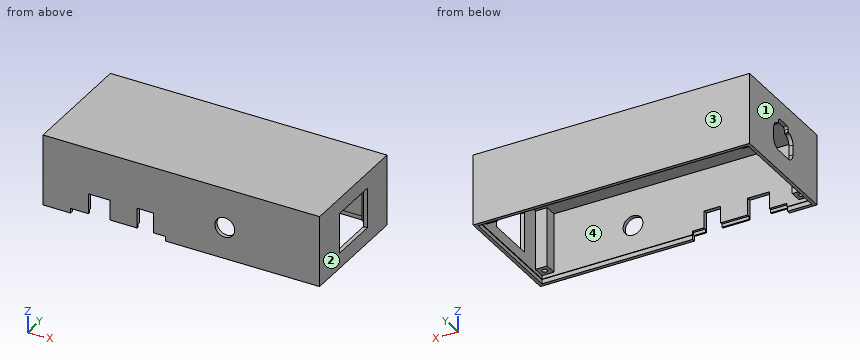
from build123d import *

# Parameters (mm, degrees)
F0_W      = 177.8
F0_H      = 76.2
F1_DEPTH  = 45.72
F2_T      = -2.54
F3_W      = 13.97
F3_H      = 16.002
F3_W_2    = 10.668
F4_DEPTH  = 2.54
F5_W      = 11.43
F5_H      = 2.54
F5_W_2    = 41.91
F5_W_3    = 7.62
F6_DEPTH  = 3.048
F8_DEPTH  = 2.54
F9_W      = 31.75
F9_H      = 25.908
F10_DEPTH = 2.54
F11_W     = 60.96
F11_H     = 1.5494
F12_DEPTH = 5.08
F13_W     = 7.62
F13_H     = 7.62
F14_DEPTH = 38.1
F15_R     = 1.5875
F16_DEPTH = 15.875
F17_R     = 6.35
F18_DEPTH = 2.54
F20_DEPTH = 2.794


with BuildPart() as f1:
    # F0 (on Top) → F1 (new body)
    with BuildSketch(Plane.XY):
        with Locations((-54.7677724445, 11.3618699834)):
            Rectangle(F0_W, F0_H)
    extrude(amount=F1_DEPTH)

    # F2
    f2_openings = [f1.faces().sort_by_distance(p)[0] for p in [
        (-54.767772, 11.36187, 0),
    ]]
    offset(amount=F2_T, openings=f2_openings)

    # F3 (on face) → F4 (cut)
    with BuildSketch(Plane.XZ.offset(26.7381300166)):
        with Locations((-107.4727724445, 8.001)):
            Rectangle(F3_W, F3_H)
        with Locations((-77.8817724445, 8.001)):
            Rectangle(F3_W_2, F3_H)
    extrude(amount=-F4_DEPTH, mode=Mode.SUBTRACT)

    # F5 (on face) → F6 (cut)
    with BuildSketch(Plane(origin=(0, 0, 0), x_dir=(1, 0, 0), z_dir=(0, 0, -1))):
        with Locations((-120.1727724445, 25.4681300166)):
            Rectangle(F5_W, F5_H)
        with Locations((-93.5027724445, 25.4681300166)):
            Rectangle(F5_W_2, F5_H)
        with Locations((-68.7377724445, 25.4681300166)):
            Rectangle(F5_W_3, F5_H)
    extrude(amount=-F6_DEPTH, mode=Mode.SUBTRACT)

    # F7 (on face) → F8 (cut)
    with BuildSketch(Plane(origin=(-143.6677724445, 0, 0), x_dir=(0, -1, 0), z_dir=(-1, 0, 0))):
        with BuildLine():
            Line((-16.6958699834, 32.385), (-16.6958699834, 30.353))
            Line((-16.6958699834, 30.353), (-6.0378982208, 30.353))
            Line((-6.0378982208, 30.353), (-5.7738699834, 30.353))
            Line((-5.7738699834, 30.353), (-5.7738699834, 32.385))
            ThreePointArc((-5.7738699834, 32.385), (-6.2202392488, 33.4626307345), (-7.2978699834, 33.909))
            Line((-7.2978699834, 33.909), (-15.1718699834, 33.909))
            ThreePointArc((-15.1718699834, 33.909), (-16.2495007179, 33.4626307345), (-16.6958699834, 32.385))
        make_face()
        with BuildLine():
            Line((-6.0378982208, 30.353), (-16.6958699834, 30.353))
            ThreePointArc((-16.6958699834, 30.353), (-20.6471826766, 28.7163126933), (-22.2838699834, 24.765))
            Line((-22.2838699834, 24.765), (-22.2838699834, 18.415))
            ThreePointArc((-22.2838699834, 18.415), (-20.6471826766, 14.4636873067), (-16.6958699834, 12.827))
            Line((-16.6958699834, 12.827), (-6.0278699834, 12.827))
            ThreePointArc((-6.0278699834, 12.827), (-2.0765572901, 14.4636873067), (-0.4398699834, 18.415))
            Line((-0.4398699834, 18.415), (-0.4398699834, 24.765))
            ThreePointArc((-0.4398699834, 24.765), (-1.5576455077, 28.1180340196), (-4.4637916501, 30.1296437876))
            Line((-4.4637916501, 30.1296437876), (-5.7738699834, 30.353))
            Line((-5.7738699834, 30.353), (-6.0378982208, 30.353))
        make_face()
    extrude(amount=-F8_DEPTH, mode=Mode.SUBTRACT)

    # F9 (on face) → F10 (cut)
    with BuildSketch(Plane.YZ.offset(34.1322275555)):
        with Locations((11.3618699834, 22.86)):
            Rectangle(F9_W, F9_H)
    extrude(amount=-F10_DEPTH, mode=Mode.SUBTRACT)

    # F11 (on face) → F12 (cut)
    with BuildSketch(Plane(origin=(0, 0, 0), x_dir=(1, 0, 0), z_dir=(0, 0, -1))):
        with Locations((-95.4077724445, 24.9728300166)):
            Rectangle(F11_W, F11_H)
    extrude(amount=-F12_DEPTH, mode=Mode.SUBTRACT)

    # F13 (on face) → F14 (join)
    with BuildSketch(Plane(origin=(0, 0, 43.18), x_dir=(1, 0, 0), z_dir=(0, 0, -1))):
        with Locations((27.7822275555, 20.3881300166)):
            Rectangle(F13_W, F13_H)
        with Locations((27.7822275555, -43.1118699834)):
            Rectangle(F13_W, F13_H)
        with Locations((-137.3177724445, 20.3881300166)):
            Rectangle(F13_W, F13_H)
        with Locations((-137.3177724445, -43.1118699834)):
            Rectangle(F13_W, F13_H)
    extrude(amount=F14_DEPTH)

    # F15 (on face) → F16 (cut)
    with BuildSketch(Plane(origin=(0, 0, 5.08), x_dir=(1, 0, 0), z_dir=(0, 0, -1))):
        with Locations((-137.3177724445, 20.3881300166)):
            Circle(F15_R)
        with Locations((-137.3177724445, -43.1118699834)):
            Circle(F15_R)
        with Locations((27.7822275555, 20.3881300166)):
            Circle(F15_R)
        with Locations((27.7822275555, -43.1118699834)):
            Circle(F15_R)
    extrude(amount=-F16_DEPTH, mode=Mode.SUBTRACT)

    # F17 (on face) → F18 (cut)
    with BuildSketch(Plane.XZ.offset(26.7381300166)):
        with Locations((-26.8277724445, 20.32)):
            Circle(F17_R)
    extrude(amount=-F18_DEPTH, mode=Mode.SUBTRACT)

    # F19 (on face) → F20 (cut)
    with BuildSketch(Plane(origin=(0, 0, 0), x_dir=(1, 0, 0), z_dir=(0, 0, -1))):
        Polygon((-125.8877724445, 24.5791300166), (-141.5087724445, 24.5791300166), (-141.5087724445, -47.3028699834), (31.9732275555, -47.3028699834), (31.9732275555, 24.5791300166), (-64.9277724445, 24.5791300166), (-64.9277724445, 24.1981300166), (31.5922275555, 24.1981300166), (31.5922275555, -46.9218699834), (-141.1277724445, -46.9218699834), (-141.1277724445, 24.1981300166), (-125.8877724445, 24.1981300166), align=None)
    extrude(amount=-F20_DEPTH, mode=Mode.SUBTRACT)


solid = f1.part
Here's how the part is built. I have some questions about the finished solid (model axes, mm). Face numbers are marked on the shaded views. Round coordinates to 2 decimals unless told otherwise and drop trailing zeros. Write each loop counter-clockwise with the first axis right and the second up, starting at its lowest first coordinate (ties: lowest second). Pieces come first, ordered by that corner, then holes.
1. Suppose I cut it at B-B (y = 34.5). List the corners of the cut face in (x, z) for me, and give its area (3 significant figures).
2. Suppose I cut it at A-A (x = 9.5). List the corners of the cut face in (y, z) for me.
3. Will these pins go through, and if not, where does the flat tip stop? pin 1 Ø4 at (x, y) = (-137, 43.5) entering from -Z; pin 2 Ø1.7 at (x, y) = (-121, -25) entering from -Z; pin 3 Ø1 at (x, y) = (6, 32.5) entering from -Z; pin 4 Ø1.3 at (x, y) = (-143, 12.5) entering from -Z.
4. I need wall thicknesses on L1, parallel to X at y = 43, z = 5.5; L2, parallel to X at y = 6.5, z = 40; L3, parallel to Y at x = -120, z = 32.5. Which ranges of each line are inside material? Lowest first, please.
5. If we mould it in two halves opening along X, with no side actions, what happens to the marked faces 1, 2, 3 and 4? For each: released by +X, released by -X, zero draft, split by the parting line, or undercut.
Answer sheet:
1. outline: (-143.67, 0) - (-141.51, 0) - (-141.51, 2.79) - (-141.13, 2.79) - (-141.13, 43.18) - (31.59, 43.18) - (31.59, 2.79) - (31.97, 2.79) - (31.97, 0) - (34.13, 0) - (34.13, 45.72) - (-143.67, 45.72) - close
1. area: 669 mm2
2. outline: (-26.74, 0) - (-24.58, 0) - (-24.58, 2.79) - (-24.2, 2.79) - (-24.2, 43.18) - (46.92, 43.18) - (46.92, 2.79) - (47.3, 2.79) - (47.3, 0) - (49.46, 0) - (49.46, 45.72) - (-26.74, 45.72) - close
3. pin 1: stops at z = 5.08
3. pin 2: stops at z = 3.05
3. pin 3: stops at z = 43.18
3. pin 4: stops at z = 0
4. L1: x = -143.67 to -138.9, -135.73 to -133.51, 23.97 to 26.2, 29.37 to 34.13
4. L2: x = -143.67 to -141.13, 31.59 to 34.13
4. L3: y = -26.74 to -24.2, 46.92 to 49.46
5. face 1: released by -X
5. face 2: released by +X
5. face 3: zero draft
5. face 4: undercut
